from build123d import *

# Parameters (mm, degrees)
SKETCH2_W           = 225.601042676
SKETCH2_H           = 112.148495204
BOSS_EXTRUDE1_DEPTH = 10
SKETCH3_R           = 5
CUT_EXTRUDE1_DEPTH  = 127.365655375


with BuildPart() as part:
    # Sketch2 → Boss-Extrude1 (new body)
    with BuildSketch(Plane(origin=(0, 0, 0), x_dir=(1, 0, 0), z_dir=(0, 1, 0))):
        Rectangle(SKETCH2_W, SKETCH2_H)
    extrude(amount=BOSS_EXTRUDE1_DEPTH)

    # Sketch3 → Cut-Extrude1 (cut, through all)
    with BuildSketch(Plane(origin=(0, 10, 0), x_dir=(1, 0, 0), z_dir=(0, 1, 0))):
        with Locations(Location((47.181724175, -18.701420381, 0), (0, 0, 270))):
            Circle(SKETCH3_R)
        with Locations(Location((47.224119262, 11.298549663, 0), (0, 0, 270))):
            Circle(SKETCH3_R)
        with Locations(Location((-42.772257947, 13.925732428, 0), (0, 0, 270))):
            Circle(SKETCH3_R)
        with Locations(Location((-62.772237976, 13.953995819, 0), (0, 0, 270))):
            Circle(SKETCH3_R)
        with Locations(Location((-62.800501368, -6.04598421, 0), (0, 0, 270))):
            Circle(SKETCH3_R)
        with Locations(Location((-62.828764759, -26.04596424, 0), (0, 0, 270))):
            Circle(SKETCH3_R)
        with Locations(Location((-42.800521338, -6.074247602, 0), (0, 0, 270))):
            Circle(SKETCH3_R)
        with Locations(Location((-42.82878473, -26.074227631, 0), (0, 0, 270))):
            Circle(SKETCH3_R)
        Polygon((-12.761689131, 21.383329852), (27.238270928, 21.326803069), (27.217073385, 6.326818047), (-12.782886674, 6.38334483), align=None)
        with BuildLine():
            Line((24.664082022, -31.169611585), (-10.33588303, -31.12015065))
            ThreePointArc((-10.33588303, -31.12015065), (-15.328812189, -26.113089794), (-10.321751334, -21.120160635))
            Line((-10.321751334, -21.120160635), (24.678213718, -21.16962157))
            ThreePointArc((24.678213718, -21.16962157), (29.671142877, -26.176682425), (24.664082022, -31.169611585))
        make_face()
    extrude(amount=-CUT_EXTRUDE1_DEPTH, mode=Mode.SUBTRACT)


solid = part.part
The listing builds one solid part. Answer for the finished solid, in the listing's coordinates (mm). A direction names the side the tool comes from. Give positions to 0.01 mm unless a question says otherwise; leave off trailing zeros. Loops run counter-clockwise (first coordinate to the right, second up) from the corner with the lowest first, then second, coordinate; pieces in that order, holes last. Notation, with made-up numbers: (-16.5, 7) - (13.5, 7) arc R22 cw to (13.5, 42) - close; hole circle Ø1 at (20.5, 51). An arc over 180 degrees is marked (long way). Use one line per item in the form item = value.
1. Find the intervals of material crossed by line 1 along Z through (x, y) = (24, 7); line 2 along Z through (x, y) = (-3.5, 1.5); line 3 along Z through (x, y) = (-39.5, 8.5), in increasing order. Write a range as [from, to].
Calculated:
line_1 = [-56.07, -21.33], [-6.33, 21.17], [31.17, 56.07]
line_2 = [-56.07, -21.37], [-6.37, 21.13], [31.13, 56.07]
line_3 = [-56.07, -17.71], [-10.15, 2.32], [9.83, 22.34], [29.81, 56.07]
2. Which of the six approach directions +Z, -Z, +X, -X, +Y, -Y give full straight-line access (tool end or side, diameter ignored) to faces 4 (the face through (-2, 10, -1)), 5 (the face through (-15.328, 5.07, 26.223))?
Calculated:
face_4 = +Z, -Z, +X, -X, +Y
face_5 = +Y, -Y
3. Section B-B on z = 26 is taken. Give the vertices of the cut face in (x, y), then the cut area to 3 significant figures.
Calculated:
outline = (-112.8, 0) - (-67.83, 0) - (-67.83, 10) - (-112.8, 10) - close; (-57.83, 0) - (-47.83, 0) - (-47.83, 10) - (-57.83, 10) - close; (-37.83, 0) - (-15.33, 0) - (-15.33, 10) - (-37.83, 10) - close; (29.67, 0) - (112.8, 0) - (112.8, 10) - (29.67, 10) - close
area = 1,610 mm^2
4. Given pin 1 Ø6 at (x, z) = (-42.83, 26.07) entering from -Y, flat-ended and moving along its own axis, determine where the tip first touches the part or whether it passes through.
Calculated:
pin_1 = through
5. Section C-C on z = -12 is taken. Give the vertices of the cut face in (x, y), then the cut area to 3 significant figures.
Calculated:
outline = (-112.8, 0) - (-67.37, 0) - (-67.37, 10) - (-112.8, 10) - close; (-58.17, 0) - (-47.39, 0) - (-47.39, 10) - (-58.17, 10) - close; (-38.16, 0) - (-12.77, 0) - (-12.77, 10) - (-38.16, 10) - close; (27.23, 0) - (42.27, 0) - (42.27, 10) - (27.23, 10) - close; (52.17, 0) - (112.8, 0) - (112.8, 10) - (52.17, 10) - close
area = 1,570 mm^2
6. Section A-A on x = -6 is taken. Give the vertices of the cut face in (y, z), then the cut area to 3 significant figures.
Calculated:
outline = (0, -56.07) - (10, -56.07) - (10, -21.37) - (0, -21.37) - close; (0, -6.37) - (10, -6.37) - (10, 21.13) - (0, 21.13) - close; (0, 31.13) - (10, 31.13) - (10, 56.07) - (0, 56.07) - close
area = 871 mm^2
7. The mould has two halves that part along X. Classify faces 1 (the face through (-2, 5, 56.074)), 2 (the face through (-112.801, 5, 1)), 3 (the face through (42.343, 5.07, -12.382)): pulls with the +X half, pulls with the -X half, needs draft (parallel to the pull), parting line crosses it, or undercut.
Calculated:
face_1 = needs draft
face_2 = pulls with the -X half
face_3 = undercut
8. Section D-D on y = 8 is taken. Count the separate pieces of the cut face and the enclosed holes in it, then the cut area to 3 significant figures.
Calculated:
separate_pieces = 1
enclosed_holes = 10
area = 23,600 mm^2
